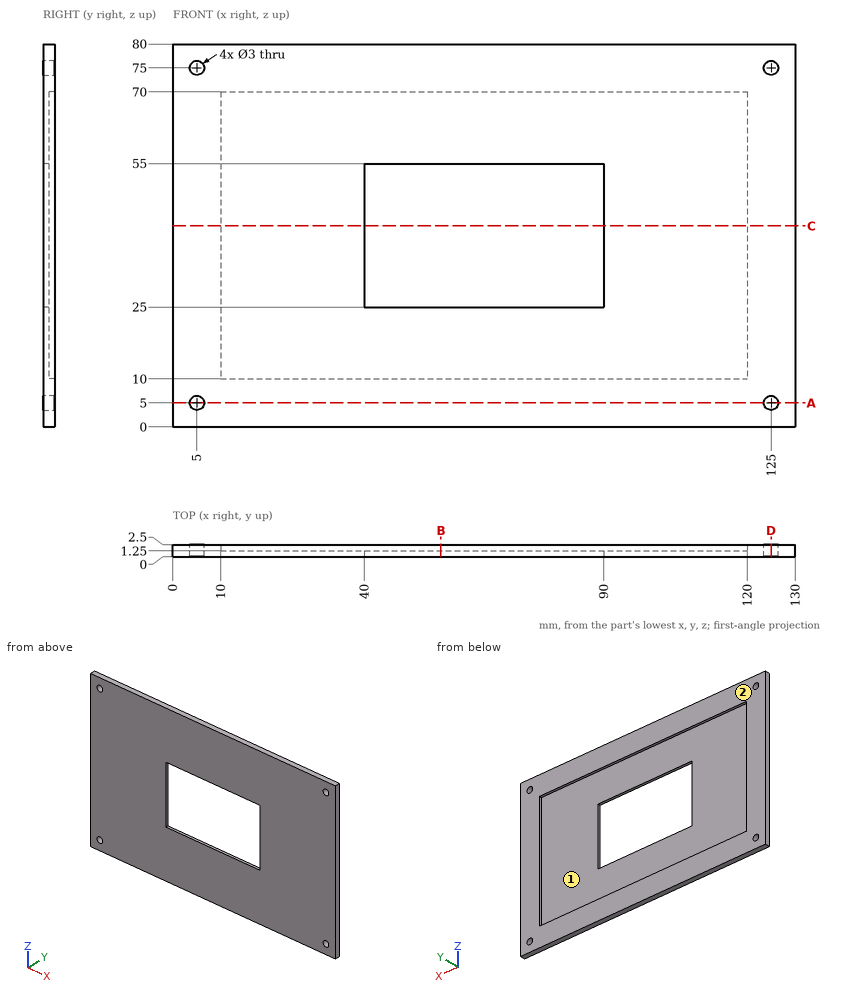
The drawing under review shows one solid part. Ordinate dimensions are in mm from its lowest x, y, z. Coordinates: 2 decimals unless noted, no trailing zeros. Write each loop counter-clockwise with the first axis right and the second up, starting at its lowest first coordinate (ties: lowest second). Pieces come first, ordered by that corner, then holes. Notation, with made-up numbers: (69, -27.5) -> (127, -27.5) arc R32 cw to (127, 0.5) -> close; hole circle Ø2 at (47.5, 79.25). An arc over 180 degrees is marked (long way). One line per item, written item: value. Start each with the question number.
Q1. Add section B-B, the plane x = 56. Give the boundary of the cut face in (y, z).
Q2. Clearance check with flat-ended pins moving along their axes: P1, Ø5, axis at x = 5, z = 75, coming from the -Y side; P2, Ø8, axis at x = 93, z = 40, coming from the +Y side. State where each tip first meets the part, or that it passes through.
Q3. Add section D-D, the plane x = 125. Give the boundary of the cut face in (y, z).
Q4. To check wall thickness, follow probe 1 along X at (y, z) = (1.5, 75); probe 2 along Z at (x, y) = (125, 1.1); probe 3 along X at (y, z) = (0.5, 36.5). State the ranges of each line that lie inside material, in increasing order.
Q5. Add section A-A, the plane z = 5. Give the boundary of the cut face in (x, y), then the cut area to 3 significant figures.
Q6. The part is to be moulded in two halves that separate along Z. For the marked faces 1 and 2, say which applies: +Z half, -Z half, draft (parallel to the pull), parting line (faces both ways), or undercut.
Q7. Add section C-C, the plane z = 42. Give the boundary of the cut face in (x, y).
Response:
1. outline: (0, 0) -> (2.5, 0) -> (2.5, 10) -> (1.25, 10) -> (1.25, 25) -> (0, 25) -> close; (0, 55) -> (1.25, 55) -> (1.25, 70) -> (2.5, 70) -> (2.5, 80) -> (0, 80) -> close
2. P1: y = 0
2. P2: y = 1.25
3. outline: (0, 0) -> (2.5, 0) -> (2.5, 3.5) -> (0, 3.5) -> close; (0, 6.5) -> (2.5, 6.5) -> (2.5, 73.5) -> (0, 73.5) -> close; (0, 76.5) -> (2.5, 76.5) -> (2.5, 80) -> (0, 80) -> close
4. probe 1: 0 to 3.5, 6.5 to 123.5, 126.5 to 130
4. probe 2: 0 to 3.5, 6.5 to 73.5, 76.5 to 80
4. probe 3: 0 to 40, 90 to 130
5. outline: (0, 0) -> (3.5, 0) -> (3.5, 2.5) -> (0, 2.5) -> close; (6.5, 0) -> (123.5, 0) -> (123.5, 2.5) -> (6.5, 2.5) -> close; (126.5, 0) -> (130, 0) -> (130, 2.5) -> (126.5, 2.5) -> close
5. area: 310 mm²
6. face 1: undercut
6. face 2: draft
7. outline: (0, 0) -> (40, 0) -> (40, 1.25) -> (10, 1.25) -> (10, 2.5) -> (0, 2.5) -> close; (90, 0) -> (130, 0) -> (130, 2.5) -> (120, 2.5) -> (120, 1.25) -> (90, 1.25) -> close
